CAD build for the part. Positions are in the model's coordinates, mm. A direction names the side the tool comes from. Give positions to 0.01 mm unless a question says otherwise; leave off trailing zeros. Loops run counter-clockwise (first coordinate to the right, second up) from the corner with the lowest first, then second, coordinate; pieces in that order, holes last.
```python
from build123d import *

# Parameters (mm, degrees)
SKETCH_1_R      = 10.5
EXTRUDE_1_DEPTH = 170
SKETCH_2_R      = 23.5
SKETCH_2_R_2    = 2
EXTRUDE_2_DEPTH = 5
EXTRUDE_START   = 5
SKETCH_3_R      = 23.5
SKETCH_3_R_2    = 2
EXTRUDE_3_DEPTH = 5


with BuildPart() as part:
    # 草图1 → 凸台-拉伸1 (new body)
    with BuildSketch(Plane.XY):
        Circle(SKETCH_1_R)
    extrude(amount=EXTRUDE_1_DEPTH)

    # 草图2 → 凸台-拉伸2 (add)
    with BuildSketch(Plane.XY.offset(170)):
        Circle(SKETCH_2_R)
        with Locations((0, 18)):
            Circle(SKETCH_2_R_2, mode=Mode.SUBTRACT)
        with Locations((-15.588457268, -9)):
            Circle(SKETCH_2_R_2, mode=Mode.SUBTRACT)
        with Locations((15.588457268, -9)):
            Circle(SKETCH_2_R_2, mode=Mode.SUBTRACT)
    extrude(amount=EXTRUDE_2_DEPTH)

    # 草图3 → 凸台-拉伸3 (add)
    with BuildSketch(Plane(origin=(0, 0, 0), x_dir=(-1, 0, 0), z_dir=(0, 0, -1)).offset(EXTRUDE_START)):
        with Locations(Location((0, 0, 0), (0, 0, 180))):
            Circle(SKETCH_3_R)
        with Locations(Location((0, 18, 0), (0, 0, 180))):
            Circle(SKETCH_3_R_2, mode=Mode.SUBTRACT)
        with Locations(Location((15.588457268, -9, 0), (0, 0, 180))):
            Circle(SKETCH_3_R_2, mode=Mode.SUBTRACT)
        with Locations(Location((-15.588457268, -9, 0), (0, 0, 180))):
            Circle(SKETCH_3_R_2, mode=Mode.SUBTRACT)
    extrude(amount=-EXTRUDE_3_DEPTH)


solid = part.part
```
1. Pull direction Z, two halves, no side cores. Call faces 3 (the face through (-17.063, -10.352, -2.535)), 4 (the face through (0, 11, 170)), 5 (the face through (0, 0, -5)): released by +Z, released by -Z, zero draft, split by the parting line, or undercut.
Responses:
face 3: zero draft
face 4: undercut
face 5: released by -Z
2. Tool access for faces 1 (the face through (14.114, -10.352, -2.535)), 2 (the face through (5, 10, 0)): list every direction of +Z, -Z, +X, -X, +Y, -Y with a clear straight run to the whole face (end or side of a thin tool).
Responses:
face 1: +Z, -Z
face 2: none
3. Probe line 1 along Z through (x, y) = (18.5, -7); line 2 along Y through (x, z) = (0, -2.1); line 3 along X through (y, z) = (-9, -3.85). List the from-to ranges inside material, lowest first.
Responses:
line 1: z = -5 to 0, 170 to 175
line 2: y = -23.5 to 16, 20 to 23.5
line 3: x = -21.71 to -17.59, -13.59 to 13.59, 17.59 to 21.71
4. Drop flat-ended pins along their axis: pin 1 (8 mm diameter, centred on y = 10, z = 154.5, fed in from -X); pin 2 (3 mm diameter, centred on y = 3, z = 84.5, fed in from +X); pin 3 (3 mm diameter, centred on y = -4.5, z = 40, fed in from +X). Give the stop position or say it passes through.
Responses:
pin 1: stops at x = -8.62
pin 2: stops at x = 10.39
pin 3: stops at x = 10.06
5. Saw through at B-B, the plane y = 0. List the corners of the cut face in (x, z), and give its area (3 significant figures).
Responses:
outline: (-23.5, -5) - (23.5, -5) - (23.5, 0) - (10.5, 0) - (10.5, 170) - (23.5, 170) - (23.5, 175) - (-23.5, 175) - (-23.5, 170) - (-10.5, 170) - (-10.5, 0) - (-23.5, 0) - close
area: 4,040 mm2
6. Saw through at D-D, the plane x = -20. List the corners of the cut face in (y, z).
Responses:
outline: (-12.34, -5) - (12.34, -5) - (12.34, 0) - (-12.34, 0) - close; (-12.34, 170) - (12.34, 170) - (12.34, 175) - (-12.34, 175) - close
7. Saw through at C-C, the plane y = -13. List the corners of the cut face in (x, z).
Responses:
outline: (-19.58, -5) - (19.58, -5) - (19.58, 0) - (-19.58, 0) - close; (-19.58, 170) - (19.58, 170) - (19.58, 175) - (-19.58, 175) - close
8. Saw through at A-A, the plane x = 0. List the corners of the cut face in (y, z), and give its area (3 significant figures).
Responses:
outline: (-23.5, -5) - (16, -5) - (16, 0) - (10.5, 0) - (10.5, 170) - (16, 170) - (16, 175) - (-23.5, 175) - (-23.5, 170) - (-10.5, 170) - (-10.5, 0) - (-23.5, 0) - close; (20, -5) - (23.5, -5) - (23.5, 0) - (20, 0) - close; (20, 170) - (23.5, 170) - (23.5, 175) - (20, 175) - close
area: 4,000 mm2
